Can you work these out from the drawing? Everything is in mm from the part's minimum corner. Coordinates: 2 decimals unless noted, no trailing zeros. Loops run counter-clockwise (first coordinate to the right, second up) from the corner with the lowest first, then second, coordinate; pieces in that order, holes last. Notation, with made-up numbers: (44, 34.5) - (103, 34.5) arc R19 ccw to (103, 57.5) - close; hole circle Ø4 at (75.25, 85). An arc over 180 degrees is marked (long way). Use CSV: the item, a comma, the result in double quotes.
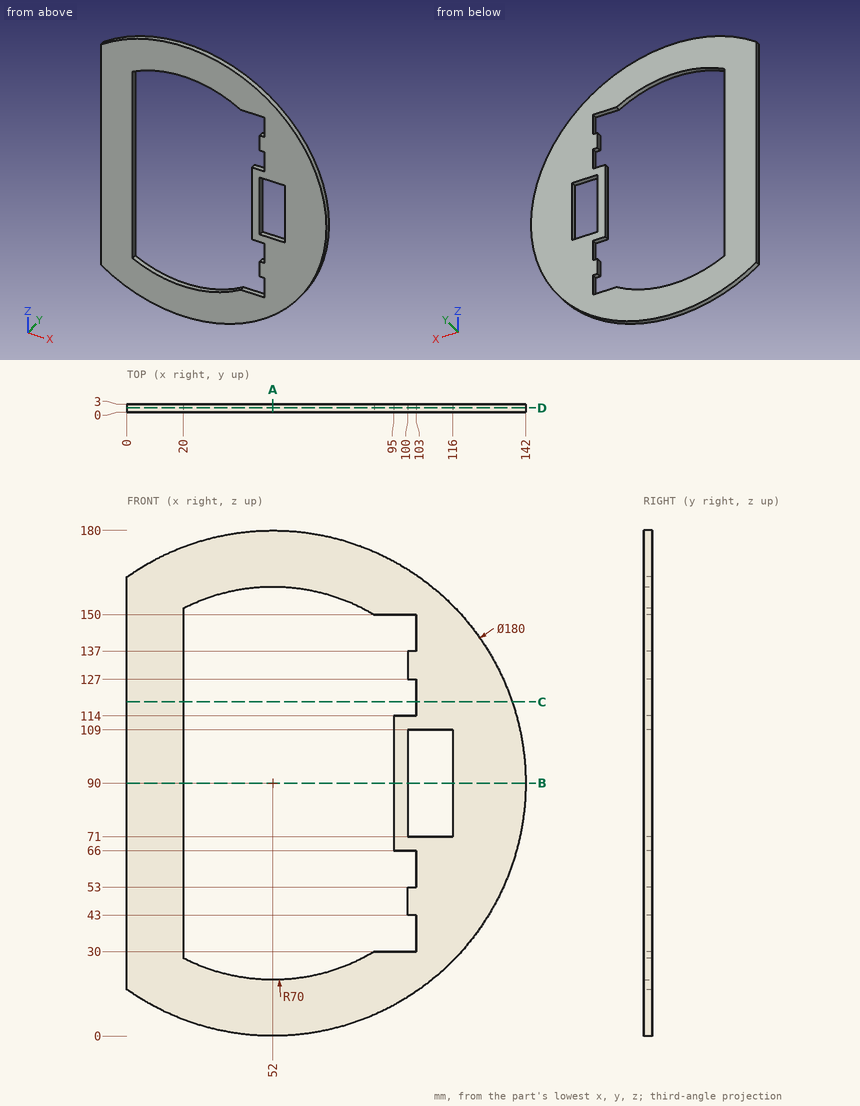
(1) Suppose I cut it at C-C (z = 119). Write out the boundary of the cut face in (x, y), plus the area to 3 significant figures.
Computed:
outline,"(0, 0) - (20, 0) - (20, 3) - (0, 3) - close; (103, 0) - (137.2, 0) - (137.2, 3) - (103, 3) - close"
area,"163 mm²"
(2) Will these pins go through, and if not, where does the flat tip stop? pin 1 (8 mm diameter, centred on x = 69.5, z = 149.5, fed in from -Y); pin 2 (1.5 mm diameter, centred on x = 99.5, y = 2, fed in from -Z); pin 3 (1.5 mm diameter, centred on x = 106.5, y = 2, fed in from -Z); pin 4 (1.5 mm diameter, centred on x = 97, y = 1, fed in from +Z).
Computed:
pin 1,"passes through"
pin 2,"stops at z = 13.09"
pin 3,"stops at z = 17.81"
pin 4,"stops at z = 168.37"
(3) Suppose I cut it at B-B (z = 90). Write out the boundary of the cut face in (x, y), plus the area to 3 significant figures.
Computed:
outline,"(0, 0) - (20, 0) - (20, 3) - (0, 3) - close; (95, 0) - (100, 0) - (100, 3) - (95, 3) - close; (116, 0) - (142, 0) - (142, 3) - (116, 3) - close"
area,"153 mm²"
(4) Suppose I cut it at D-D (y = 1.65). Write out the boundary of the cut face in (x, z), plus the area to 3 significant figures.
Computed:
outline,"(0, 16.54) arc R90 ccw (long way) to (0, 163.46) - close; hole (20, 27.74) arc R70 ccw to (88.06, 30) - (103, 30) - (103, 43) - (100, 43) - (100, 53) - (103, 53) - (103, 66) - (95, 66) - (95, 114) - (103, 114) - (103, 127) - (100, 127) - (100, 137) - (103, 137) - (103, 150) - (88.06, 150) arc R70 ccw to (20, 152.26) - close; hole (100, 71) - (116, 71) - (116, 109) - (100, 109) - close"
area,"10,400 mm²"
(5) Suppose I cut it at A-A (x = 52). Write out the boundary of the cut face in (y, z), plus the area to 3 significant figures.
Computed:
outline,"(0, 0) - (3, 0) - (3, 20) - (0, 20) - close; (0, 160) - (3, 160) - (3, 180) - (0, 180) - close"
area,"120 mm²"
(6) Please list where these lines run through material, in increasing order: line 1 (Z direction, x = 97, y = 0.85); line 2 (X direction, y = 1, z = 99); line 3 (Z direction, x = 51, y = 2.35).
Computed:
line 1,"z = 12.06 to 30, 66 to 114, 150 to 167.94"
line 2,"x = 0 to 20, 95 to 100, 116 to 141.55"
line 3,"z = 0.01 to 20.01, 159.99 to 179.99"
